Model file for the job. Use its own axes, mm. A direction names the side the tool comes from. Round coordinates to 2 decimals unless told otherwise and drop trailing zeros. Loops run counter-clockwise (first coordinate to the right, second up) from the corner with the lowest first, then second, coordinate; pieces in that order, holes last. Notation, with made-up numbers: M 79,31 L 121,31 A34 cw 121,61 Z; hole C 14.5,-39.75 d11. An arc over 180 degrees is marked long. Use a Markdown table: item, result. Add a question column.
Q1. Pin check, flat tips, straight feed: pin 1 (3 mm diameter, centred on y = 7.5, z = 4.5, fed in from +X); pin 2 (0.8 mm diameter, centred on x = 22, y = 1, fed in from +Z); pin 3 (5 mm diameter, centred on x = -45.5, y = 7.5, fed in from +Z). Stop position of each tip, or through.
Q2. Cut at B-B (z = 18). Give the cut face in (x, y).
Q3. Cut at A-A (y = 9.25). Give the cut face in (x, z), plus the area to 4 significant figures.
Q4. Probe line 1 (Z direction, x = 50, y = 1); line 2 (X direction, y = 1.35, z = -40); line 3 (Z direction, x = 47, y = 3.5). List the from-to ranges inside material, lowest first. Write a range as from..to.
Q5. Tool access for faces 1 (the face through (-33, 7, 35.75)), 2 (the face through (49, 7, 8)), 3 (the face through (49, 7, 13)): list every direction of +Z, -Z, +X, -X, +Y, -Y with a clear straight run to the whole face (end or side of a thin tool).
Q6. Mould opens along X. For faces 4 (the face through (53, 1, -44)), 5 (the face through (44.5, 7, 23)), 6 (the face through (-33, 1.7, 48)) say: +X half, -X half, draft (parallel to the pull), parting line (faces both ways), or undercut.
Q7. Cut at C-C (x = 28). Give the cut face in (y, z), plus the area to 3 significant figures.
Q8. Cut at D-D (z = 31.5). Give the cut face in (x, y).
from build123d import *

# Parameters (mm, degrees)
SKETCH1_W                      = 110
SKETCH1_H                      = 90
BOSS_EXTRUDE1_DEPTH            = 1.7
CUT_EXTRUDE1_REACH             = 3.7
SKETCH2_R                      = 1.75
CUT_EXTRUDE1_DIRECTION_2_DEPTH = 1
FILLET1_R                      = 5
SKETCH3_W                      = 10.5
SKETCH3_H                      = 10.5
BOSS_EXTRUDE2_DEPTH            = 18
CHAMFER1_SIZE                  = 5
SKETCH4_W                      = 12
SKETCH4_H                      = 16.25
BOSS_EXTRUDE3_DEPTH            = 11
SKETCH5_W                      = 9
SKETCH5_H                      = 20
BOSS_EXTRUDE4_DEPTH            = 10


with BuildPart() as part:
    # Sketch1 → Boss-Extrude1 (new body)
    with BuildSketch(Plane(origin=(0, 0, 0), x_dir=(1, 0, 0), z_dir=(0, 1, 0))):
        Rectangle(SKETCH1_W, SKETCH1_H)
    extrude(amount=BOSS_EXTRUDE1_DEPTH)

    # Sketch2 → Cut-Extrude1 (cut, up to next)
    with BuildSketch(Plane(origin=(0, 1.7, 0), x_dir=(1, 0, 0), z_dir=(0, 1, 0)), mode=Mode.PRIVATE) as cut_extrude1_sk1:
        with Locations((-50, 40)):
            Circle(SKETCH2_R)
    cut_extrude1_tool1 = extrude(cut_extrude1_sk1.sketch, amount=-CUT_EXTRUDE1_REACH, mode=Mode.PRIVATE) & part.part
    add(cut_extrude1_tool1.solids().sort_by_distance((-50, 1.7, -40))[0], mode=Mode.SUBTRACT)
    # Sketch2 → Cut-Extrude1 (cut, up to next)
    with BuildSketch(Plane(origin=(0, 1.7, 0), x_dir=(1, 0, 0), z_dir=(0, 1, 0)), mode=Mode.PRIVATE) as cut_extrude1_sk2:
        with Locations((-50, -40)):
            Circle(SKETCH2_R)
    cut_extrude1_tool2 = extrude(cut_extrude1_sk2.sketch, amount=-CUT_EXTRUDE1_REACH, mode=Mode.PRIVATE) & part.part
    add(cut_extrude1_tool2.solids().sort_by_distance((-50, 1.7, 40))[0], mode=Mode.SUBTRACT)
    # Sketch2 → Cut-Extrude1 (cut, up to next)
    with BuildSketch(Plane(origin=(0, 1.7, 0), x_dir=(1, 0, 0), z_dir=(0, 1, 0)), mode=Mode.PRIVATE) as cut_extrude1_sk3:
        with Locations((50, -40)):
            Circle(SKETCH2_R)
    cut_extrude1_tool3 = extrude(cut_extrude1_sk3.sketch, amount=-CUT_EXTRUDE1_REACH, mode=Mode.PRIVATE) & part.part
    add(cut_extrude1_tool3.solids().sort_by_distance((50, 1.7, 40))[0], mode=Mode.SUBTRACT)
    # Sketch2 → Cut-Extrude1 (cut, up to next)
    with BuildSketch(Plane(origin=(0, 1.7, 0), x_dir=(1, 0, 0), z_dir=(0, 1, 0)), mode=Mode.PRIVATE) as cut_extrude1_sk4:
        with Locations((50, 40)):
            Circle(SKETCH2_R)
    cut_extrude1_tool4 = extrude(cut_extrude1_sk4.sketch, amount=-CUT_EXTRUDE1_REACH, mode=Mode.PRIVATE) & part.part
    add(cut_extrude1_tool4.solids().sort_by_distance((50, 1.7, -40))[0], mode=Mode.SUBTRACT)

    # Sketch2 → Cut-Extrude1 direction 2 (cut)
    with BuildSketch(Plane(origin=(0, 1.7, 0), x_dir=(1, 0, 0), z_dir=(0, 1, 0))):
        with Locations((-50, 40)):
            Circle(SKETCH2_R)
        with Locations((-50, -40)):
            Circle(SKETCH2_R)
        with Locations((50, -40)):
            Circle(SKETCH2_R)
        with Locations((50, 40)):
            Circle(SKETCH2_R)
    extrude(amount=CUT_EXTRUDE1_DIRECTION_2_DEPTH, mode=Mode.SUBTRACT)

    # Fillet1
    fillet1_edges = [part.edges().sort_by_distance(p)[0] for p in [
        (55, 0.85, 45),
        (-55, 0.85, 45),
        (-55, 0.85, -45),
        (55, 0.85, -45),
    ]]
    fillet(fillet1_edges, radius=FILLET1_R)

    # Sketch3 → Boss-Extrude2 (add)
    with BuildSketch(Plane(origin=(0, 1.7, 0), x_dir=(1, 0, 0), z_dir=(0, 1, 0))):
        with Locations((-46.25, -27.45)):
            Rectangle(SKETCH3_W, SKETCH3_H)
        with Locations((-46.25, -4.95)):
            Rectangle(SKETCH3_W, SKETCH3_H)
    extrude(amount=BOSS_EXTRUDE2_DEPTH)

    # Chamfer1
    chamfer1_edges = [part.edges().sort_by_distance(p)[0] for p in [
        (-51.5, 19.7, 27.45),
        (-51.5, 19.7, 4.95),
    ]]
    chamfer(chamfer1_edges, length=CHAMFER1_SIZE)

    # Sketch4 → Boss-Extrude3 (add)
    with BuildSketch(Plane(origin=(0, 1.7, 0), x_dir=(1, 0, 0), z_dir=(0, 1, 0))):
        with Locations((-33, -43.875)):
            Rectangle(SKETCH4_W, SKETCH4_H)
    extrude(amount=BOSS_EXTRUDE3_DEPTH)

    # Sketch5 → Boss-Extrude4 (add)
    with BuildSketch(Plane(origin=(0, 1.7, 0), x_dir=(1, 0, 0), z_dir=(0, 1, 0))):
        with Locations((49, -23)):
            Rectangle(SKETCH5_W, SKETCH5_H)
        with Locations((49, 2)):
            Rectangle(SKETCH5_W, SKETCH5_H)
    extrude(amount=BOSS_EXTRUDE4_DEPTH)


solid = part.part
Checked values:
| question | item | result |
|---|---|---|
| 1 | pin 1 | stops at x = 53.5 |
| 1 | pin 2 | stops at z = 45 |
| 1 | pin 3 | stops at z = 32.7 |
| 2 | outline | M -55,0 L 55,0 L 55,1.7 L 53.5,1.7 L 53.5,11.7 L 44.5,11.7 L 44.5,1.7 L -55,1.7 Z |
| 3 | outline | M -51.5,-0.3 L -41,-0.3 L -41,10.2 L -51.5,10.2 Z; M -51.5,22.2 L -41,22.2 L -41,32.7 L -51.5,32.7 Z; M -39,35.75 L -27,35.75 L -27,52 L -39,52 Z; M 44.5,-12 L 53.5,-12 L 53.5,8 L 44.5,8 Z; M 44.5,13 L 53.5,13 L 53.5,33 L 44.5,33 Z |
| 3 | area | 775.5 mm^2 |
| 4 | line 1 | z = -45..-41.75, -38.25..38.25, 41.75..45 |
| 4 | line 2 | x = -55..-51.75, -48.25..48.25, 51.75..55 |
| 4 | line 3 | z = -12..8, 13..33 |
| 5 | face 1 | -Z, +X, -X, +Y |
| 5 | face 2 | +X, +Y |
| 5 | face 3 | +X, -X, +Y |
| 6 | face 4 | +X half |
| 6 | face 5 | undercut |
| 6 | face 6 | draft |
| 7 | outline | M 0,-45 L 1.7,-45 L 1.7,45 L 0,45 Z |
| 7 | area | 153 mm^2 |
| 8 | outline | M -55,0 L 55,0 L 55,1.7 L 53.5,1.7 L 53.5,11.7 L 44.5,11.7 L 44.5,1.7 L -41,1.7 L -41,19.7 L -46.5,19.7 L -51.5,14.7 L -51.5,1.7 L -55,1.7 Z |
